Source: CAD feature listing. Evaluate the final solid. Frame: model axes, mm. Face numbers are marked on the shaded views. A direction names the side the tool comes from. Round coordinates to 2 decimals unless told otherwise and drop trailing zeros. Write each loop counter-clockwise with the first axis right and the second up, starting at its lowest first coordinate (ties: lowest second). Pieces come first, ordered by that corner, then holes. Notation, with made-up numbers: (63, 28.5) -> (69, 28.5) arc R17 ccw to (69, 61.5) -> close; hole circle Ø1 at (37, -19.75). An arc over 180 degrees is marked (long way). Put each result on its own line as item: value.
```python
from build123d import *

# Parameters (mm, degrees)
F1_DEPTH = 12.7
F2_R     = 3.175
F3_R     = 3.81
F4_DEPTH = 25.4
F5_R     = 3.81
F6_DEPTH = 25.4


with BuildPart() as f1:
    # F0 (on Right) → F1 (new body, symmetric)
    with BuildSketch(Plane.YZ):
        Polygon((0, 6.35), (0, 0), (25.4, 0), (25.4, 25.4), (19.05, 25.4), (19.05, 6.35), align=None)
    extrude(amount=F1_DEPTH, both=True)

    # F2
    f2_edges = [f1.edges().sort_by_distance(p)[0] for p in [
        (0, 0, 6.35),
        (0, 19.05, 6.35),
        (0, 19.05, 25.4),
    ]]
    fillet(f2_edges, radius=F2_R)

    # F3 (on face) → F4 (cut)
    with BuildSketch(Plane.XY.offset(6.35)):
        with Locations((0, 9.525)):
            Circle(F3_R)
    extrude(amount=-F4_DEPTH, mode=Mode.SUBTRACT)

    # F5 (on face) → F6 (cut)
    with BuildSketch(Plane.XZ.offset(-19.05)):
        with Locations((0, 15.875)):
            Circle(F5_R)
    extrude(amount=-F6_DEPTH, mode=Mode.SUBTRACT)


solid = f1.part
```
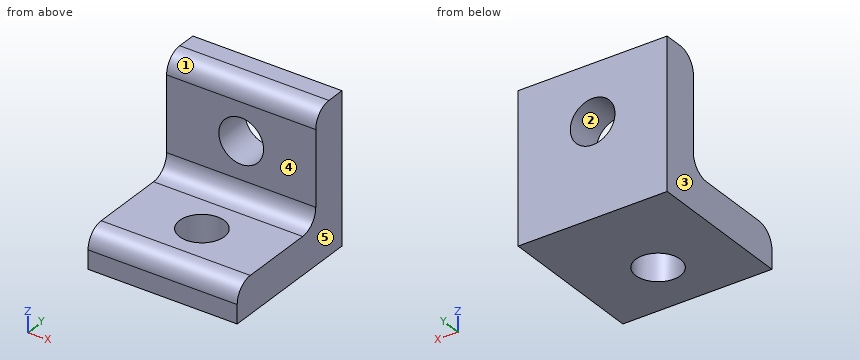
Q1. Cut plane C-C on y = 24. Output: boundary loops of the cut face in (x, z) (3 decimals), and give its area (3 significant figures).
Ans:
outline: (-12.7, 0) -> (12.7, 0) -> (12.7, 25.4) -> (-12.7, 25.4) -> close; hole circle Ø7.62 at (0, 15.875)
area: 600 mm^2
Q2. Cut plane A-A on z = 18.25. Output: boundary loops of the cut face in (x, y), and give its area (3 significant figures).
Ans:
outline: (-12.7, 19.05) -> (-2.98, 19.05) -> (-2.98, 25.4) -> (-12.7, 25.4) -> close; (2.98, 19.05) -> (12.7, 19.05) -> (12.7, 25.4) -> (2.98, 25.4) -> close
area: 123 mm^2
Q3. Reachability of the marked faces 4 and 5 from +Z, -Z, +X, -X, +Y, -Y: full face, straight path, thin tool, end or side. Return the list, or none.
Ans:
face 4: +Z, +X, -X, -Y
face 5: +Z, -Z, +X, +Y, -Y
Q4. Draft query along X for the marked faces 1, 2 and 3. Return one class per face: +X half, -X half, draft (parallel to the pull), parting line (faces both ways), or undercut.
Ans:
face 1: draft
face 2: undercut
face 3: -X half
Q5. Pin query (flat end, axial travel): pin 1 (12 mm diameter, centred on x = 0, z = 15.875, fed in from -Y); pin 2 (4.5 mm diameter, centred on x = 0, y = 9.525, fed in from +Z); pin 3 (4 mm diameter, centred on x = 8, y = 12.5, fed in from +Z); pin 4 (6 mm diameter, centred on x = 7, y = 11.5, fed in from +Z). Return the tip coordinate at first contact, or that it passes through.
Ans:
pin 1: stops at y = 19.05
pin 2: passes through
pin 3: stops at z = 6.35
pin 4: stops at z = 6.35
Q6. Cut plane D-D on x = 6.5. Output: boundary loops of the cut face in (y, z) (3 decimals), and give its area (3 significant figures).
Ans:
outline: (0, 0) -> (25.4, 0) -> (25.4, 25.4) -> (22.225, 25.4) arc R3.175 ccw to (19.05, 22.225) -> (19.05, 9.525) arc R3.175 cw to (15.875, 6.35) -> (3.175, 6.35) arc R3.175 ccw to (0, 3.175) -> close
area: 280 mm^2
Q7. Material intervals for line 1 (Y direction, x = 0, z = 3) (3 decimals); line 2 (Z direction, x = 0, y = 24) (3 decimals); line 3 (Y direction, x = -7.5, z = 18.75), sorted ascending. Write a range as [from, to].
Ans:
line 1: y = [0, 5.715], [13.335, 25.4]
line 2: z = [0, 12.065], [19.685, 25.4]
line 3: y = [19.05, 25.4]
Q8. Cut plane B-B on x = 0. Output: boundary loops of the cut face in (y, z) (3 decimals), and give its area (3 significant figures).
Ans:
outline: (0, 0) -> (5.715, 0) -> (5.715, 6.35) -> (3.175, 6.35) arc R3.175 ccw to (0, 3.175) -> close; (13.335, 0) -> (25.4, 0) -> (25.4, 12.065) -> (19.05, 12.065) -> (19.05, 9.525) arc R3.175 cw to (15.875, 6.35) -> (13.335, 6.35) -> close; (19.05, 19.685) -> (25.4, 19.685) -> (25.4, 25.4) -> (22.225, 25.4) arc R3.175 ccw to (19.05, 22.225) -> close
area: 183 mm^2
